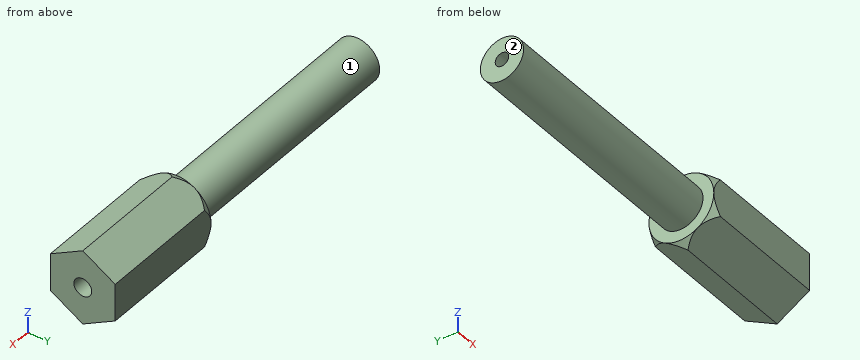
from build123d import *

# Parameters (mm, degrees)
BOSS_EXTRU_1_DEPTH        = 67.5
TROU_TARAUD_M4X0_71_D     = 3.3
TROU_TARAUD_M4X0_71_DEPTH = 15
TROU_TARAUD_M4X0_71_TIP   = 0.991420021
TROU_TARAUD_M3X0_51_D     = 2.5
TROU_TARAUD_M3X0_51_DEPTH = 15
TROU_TARAUD_M3X0_51_TIP   = 0.751075774


with BuildPart() as part:
    # Esquisse1 → Boss.-Extru.1 (new body)
    with BuildSketch(Plane(origin=(0, 0, 0), x_dir=(0, 0, -1), z_dir=(1, 0, 0))):
        Polygon((6.92820323, 0), (3.464101615, 6), (-3.464101615, 6), (-6.92820323, 0), (-3.464101615, -6), (3.464101615, -6), align=None)
    extrude(amount=-BOSS_EXTRU_1_DEPTH)

    # Trou taraudé M4x0.71
    with Locations(Plane(origin=(0, 0, 0), x_dir=(0, 0, -1), z_dir=(1, 0, 0))):
        with Locations((0, 0)):
            Hole(TROU_TARAUD_M4X0_71_D / 2, depth=TROU_TARAUD_M4X0_71_DEPTH)
            with Locations((0, 0, -(TROU_TARAUD_M4X0_71_DEPTH + TROU_TARAUD_M4X0_71_TIP / 2))):  # 118° drill point
                Cone(0, TROU_TARAUD_M4X0_71_D / 2, TROU_TARAUD_M4X0_71_TIP, mode=Mode.SUBTRACT)

    # Trou taraudé M3x0.51
    with Locations(Plane.ZY.offset(67.5)):
        with Locations((0, 0)):
            Hole(TROU_TARAUD_M3X0_51_D / 2, depth=TROU_TARAUD_M3X0_51_DEPTH)
            with Locations((0, 0, -(TROU_TARAUD_M3X0_51_DEPTH + TROU_TARAUD_M3X0_51_TIP / 2))):  # 118° drill point
                Cone(0, TROU_TARAUD_M3X0_51_D / 2, TROU_TARAUD_M3X0_51_TIP, mode=Mode.SUBTRACT)

    # Esquisse4 → Enlèvement de matière-Révolution1 (revolve, cut)
    with BuildSketch(Plane(origin=(0, 0, 0), x_dir=(1, 0, 0), z_dir=(0, 1, 0))):
        Polygon((-21.892304845, 6.92820323), (-67.5, 6.92820323), (-67.5, 4), (-23.5, 4), (-23.5, 6), align=None)
    revolve(axis=Axis((0, 0, 0), (-1, 0, 0)), mode=Mode.SUBTRACT)


solid = part.part
Source: CAD feature listing. Evaluate the final solid. Frame: model axes, mm. Face numbers are marked on the shaded views. A direction names the side the tool comes from. Give positions to 0.01 mm unless a question says otherwise; leave off trailing zeros. Write each loop counter-clockwise with the first axis right and the second up, starting at its lowest first coordinate (ties: lowest second). Pieces come first, ordered by that corner, then holes. Notation, with made-up numbers: (64.25, 72) -> (110.25, 72) arc R16 ccw to (110.25, 88) -> close; hole circle Ø4 at (23.5, 15). An arc over 180 degrees is marked (long way). Return JSON: item names as keys, results as strings. Group by question number.
1. Pin query (flat end, axial travel): pin 1 Ø2 at (y, z) = (0, 0) entering from +X; pin 2 Ø4 at (x, y) = (-9.5, 0.5) entering from -Z; pin 3 Ø5 at (x, y) = (-58.5, -3) entering from +Z. Return the tip coordinate at first contact, or that it passes through.
2. Section C-C, the plane x = -57. Output: boundary loops of the cut face in (y, z), then the cut area to 3 significant figures.
3. Access query for the marked faces 1 and 2. Directions: +Z, -Z, +X, -X, +Y, -Y. A direction counts if a zero-diameter tool reaches every point of the face in a straight line with its end or side. Return the directions, or none.
4. Section B-B, the plane x = -25. Output: boundary loops of the cut face in (y, z), then the cut area to 3 significant figures.
5. Section A-A, the plane x = -8.5. Output: boundary loops of the cut face in (y, z).
6. Material intervals for line 1 (Y direction, x = -10, z = 0); line 2 (Y direction, x = -61.5, z = 0), sorted ascending. Write a range as from..to.
Determined:
{
 "1": {"pin 1": "stops at x = -15.39", "pin 2": "stops at z = -6.93", "pin 3": "stops at z = 3.97"},
 "2": {"outline": "circle Ø8 at (0, 0); hole circle Ø2.5 at (0, 0)", "area": "45.4 mm2"},
 "3": {"face 1": "-X", "face 2": "+Z, -Z, -X, +Y, -Y"},
 "4": {"outline": "circle Ø8 at (0, 0)", "area": "50.3 mm2"},
 "5": {"outline": "(-6, -3.46) -> (0, -6.93) -> (6, -3.46) -> (6, 3.46) -> (0, 6.93) -> (-6, 3.46) -> close; hole circle Ø3.3 at (0, 0)"},
 "6": {"line 1": "y = -6..-1.65, 1.65..6", "line 2": "y = -4..-1.25, 1.25..4"}
}
